```python
from build123d import *

# Parameters (mm, degrees)
SKETCH1_W           = 111
SKETCH1_H           = 126.5
BOSS_EXTRUDE1_DEPTH = 6
SKETCH2_W           = 60
SKETCH2_H           = 80
CUT_EXTRUDE1_DEPTH  = 7
FILLET1_R           = 5


with BuildPart() as part:
    # Sketch1 → Boss-Extrude1 (new body)
    with BuildSketch(Plane(origin=(0, 0, 0), x_dir=(1, 0, 0), z_dir=(0, 1, 0))):
        with Locations((55.5, 63.25)):
            Rectangle(SKETCH1_W, SKETCH1_H)
    extrude(amount=BOSS_EXTRUDE1_DEPTH)

    # Sketch2 → Cut-Extrude1 (cut, through all)
    with BuildSketch(Plane(origin=(0, 6, 0), x_dir=(1, 0, 0), z_dir=(0, 1, 0))):
        with Locations((30, 63.25)):
            Rectangle(SKETCH2_W, SKETCH2_H)
    extrude(amount=-CUT_EXTRUDE1_DEPTH, mode=Mode.SUBTRACT)

    # Fillet1
    fillet1_edges = [part.edges().sort_by_distance(p)[0] for p in [
        (60, 3, -103.25),
        (60, 3, -23.25),
    ]]
    fillet(fillet1_edges, radius=FILLET1_R)


solid = part.part
```
Build history of the part. All positions in model axes, mm. A direction names the side the tool comes from. Coordinates: 2 decimals unless noted, no trailing zeros. Order: outer loops, then holes, each group sorted by start corner. A loop starts at its lowest first (then second) coordinate and runs counter-clockwise, first axis right, second up. Notation, with made-up numbers: (67, 13) -> (85, 13) arc R12 ccw to (85, 33) -> close; hole circle Ø10 at (85, 21.5). An arc over 180 degrees is marked (long way). Answer in a Markdown table with one row per item. Add a question column.
Q1. Wall check: line 1 along Z through (x, y) = (48, 1.35); line 2 along X through (y, z) = (4.9, -24.5). Give the ranges that are in metal, low to high. Write a range as [from, to].
Q2. Band-saw the part on A-A, the plane x = 40.5. List the corners of the cut face in (y, z).
Q3. Band-saw the part on B-B, the plane y = 1.6. List the corners of the cut face in (x, z).
Q4. Band-saw the part on C-C, the plane z = -90.5. List the corners of the cut face in (x, y).
Q5. Mould opens along Z. For faces 1 (the face through (55, 3, 0)), 2 (the face through (55, 3, -126.5)), 3 (the face through (58.5, 2.96, -24.68)), 4 (the face through (111, 3, -62)) say: +Z half, -Z half, draft (parallel to the pull), parting line (faces both ways), or undercut.
Q6. Which spindle directions (+Z, -Z, +X, -X, +Y, -Y) get a long thin tool onto all of the face, cutting with end or side? Do faces 5 (the face through (67, 6, -64)), 6 (the face through (27, 3, -23.25)). Say none if no direction does.
Answers follow:
| question | item | result |
|---|---|---|
| 1 | line 1 | [-126.5, -103.25], [-23.25, 0] |
| 1 | line 2 | [58.31, 111] |
| 2 | outline | (0, -126.5) -> (6, -126.5) -> (6, -103.25) -> (0, -103.25) -> close; (0, -23.25) -> (6, -23.25) -> (6, 0) -> (0, 0) -> close |
| 3 | outline | (0, -126.5) -> (111, -126.5) -> (111, 0) -> (0, 0) -> (0, -23.25) -> (55, -23.25) arc R5 cw to (60, -28.25) -> (60, -98.25) arc R5 cw to (55, -103.25) -> (0, -103.25) -> close |
| 4 | outline | (60, 0) -> (111, 0) -> (111, 6) -> (60, 6) -> close |
| 5 | face 1 | +Z half |
| 5 | face 2 | -Z half |
| 5 | face 3 | undercut |
| 5 | face 4 | draft |
| 6 | face 5 | +Z, -Z, +X, -X, +Y |
| 6 | face 6 | -X, +Y, -Y |
